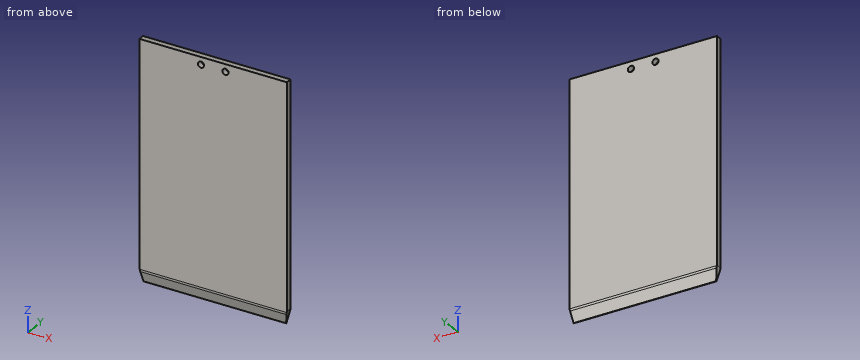
```python
from build123d import *

# Parameters (mm, degrees)
F1_DEPTH = 150
F3_DEPTH = 25


with BuildPart() as f1:
    # F0 (on Right) → F1 (new body, symmetric)
    with BuildSketch(Plane.YZ):
        with BuildLine():
            Line((6, -215.287568), (6, 242.5))
            Line((6, 242.5), (-6, 242.5))
            Line((-6, 242.5), (-6, -216.946892))
            ThreePointArc((-6, -216.946892), (-5.859226, -219.315681), (-5.438884, -221.651124))
            Line((-5.438884, -221.651124), (-0.485972, -242.117606))
            ThreePointArc((-0.485972, -242.117606), (-0.05922, -241.503519), (0.5, -242))
            ThreePointArc((0.5, -242), (0.496969, -242.054975), (0.487911, -242.109284))
            Line((0.487911, -242.109284), (5.516432, -219.658939))
            ThreePointArc((5.516432, -219.658939), (5.87874, -217.486586), (6, -215.287568))
        make_face()
        with BuildLine():
            ThreePointArc((0, -242.5), (0.312536, -242.390283), (0.487911, -242.109284))
            ThreePointArc((0.487911, -242.109284), (0.496969, -242.054975), (0.5, -242))
            ThreePointArc((0.5, -242), (-0.05922, -241.503519), (-0.485972, -242.117606))
            ThreePointArc((-0.485972, -242.117606), (-0.30919, -242.392939), (0, -242.5))
        make_face()
    extrude(amount=F1_DEPTH, both=True)

    # F2 (on face) → F3 (cut)
    with BuildSketch(Plane(origin=(0, 6, 0), x_dir=(-1, 0, 0), z_dir=(0, 1, 0))):
        with BuildLine():
            Line((18.75, 227.25), (31.25, 227.25))
            ThreePointArc((31.25, 227.25), (25, 233.5), (18.75, 227.25))
        make_face()
        with BuildLine():
            ThreePointArc((-31.25, 227.25), (-25, 221), (-18.75, 227.25))
            Line((-18.75, 227.25), (-31.25, 227.25))
        make_face()
        with BuildLine():
            Line((-31.25, 227.25), (-18.75, 227.25))
            ThreePointArc((-18.75, 227.25), (-25, 233.5), (-31.25, 227.25))
        make_face()
        with BuildLine():
            ThreePointArc((18.75, 227.25), (25, 221), (31.25, 227.25))
            Line((31.25, 227.25), (18.75, 227.25))
        make_face()
        Polygon((-145, -242.499982), (-150, -214.500172), (-150.103354, -242.499982), align=None)
        Polygon((150.103354, -242.499982), (150, -214.500172), (145, -242.499982), align=None)
    extrude(amount=-F3_DEPTH, mode=Mode.SUBTRACT)


solid = f1.part
```
Check sheet for the modelled part. Datum: model origin and axes. Units: mm. Give positions to 0.01 mm unless a question says otherwise; leave off trailing zeros. Loops run counter-clockwise (first coordinate to the right, second up) from the corner with the lowest first, then second, coordinate; pieces in that order, holes last. Notation, with made-up numbers: M 18.25,-14.75 L 67.25,-14.75 A4 ccw 67.25,-10.75 Z; hole C 61,82 d9. An arc over 180 degrees is marked long. Answer as CSV lines item,"result".
Item 1: Sectioned sample at B-B, the plane z = 227.25. Enter the section's corners in (x, y), then the cut area to 3 significant figures.
Reply:
outline,"M -150,-6 L -31.25,-6 L -31.25,6 L -150,6 Z; M -18.75,-6 L 18.75,-6 L 18.75,6 L -18.75,6 Z; M 31.25,-6 L 150,-6 L 150,6 L 31.25,6 Z"
area,"3,300 mm^2"
Item 2: Scan line: L1, parallel to Z at x = -25, y = 0.25. Record every from-to range of solid material in increasing order.
Reply:
L1,"-242.43 to 221, 233.5 to 242.5"
Item 3: Depth check by flat-ended pin: pin 1 Ø16 at (x, z) = (25, 227.25) entering from +Y. Enter the tip coordinate at first touch or a pass-through.
Reply:
pin 1,"y = 6"
Item 4: Sectioned sample at C-C, the plane y = -2.5. Enter the section's corners in (x, z), then the cut area to 3 significant figures.
Reply:
outline,"M -150,-214.5 L -146.55,-233.8 L 146.55,-233.8 L 150,-214.5 L 150,242.5 L -150,242.5 Z; hole C -25,227.25 d12.5; hole C 25,227.25 d12.5"
area,"143,000 mm^2"
Item 5: Sectioned sample at A-A, the plane x = -25. Enter the section's corners in (y, z).
Reply:
outline,"M -6,-216.95 A20 ccw -5.44,-221.65 L -0.49,-242.12 A0.5 ccw 0,-242.5 A0.5 ccw 0.49,-242.11 L 5.52,-219.66 A20 ccw 6,-215.29 L 6,221 L -6,221 Z; M -6,233.5 L 6,233.5 L 6,242.5 L -6,242.5 Z"
